Could you check a few things on this model? Use its own coordinates, in mm. A direction names the side the tool comes from. Coordinates: 2 decimals unless noted, no trailing zeros. Write each loop counter-clockwise with the first axis right and the second up, starting at its lowest first coordinate (ties: lowest second). Pieces come first, ordered by that corner, then holes. Notation, with made-up numbers: (36, -34) - (71, -34) arc R30 ccw to (71, 2) - close; hole circle Ø2 at (60.25, 39). An arc over 180 degrees is marked (long way). Answer as a JSON object with one key per item and string values. Group by question number.
1) On a 3-axis mill with a long thin cutter (end or side, diameter ignored), from which of +Z, -Z, +X, -X, +Y, -Y can I reach the whole of each face in a straight line? I mean faces 4 (the flat face through (0, -19, 12)), 5 (the flat face through (19, 0, 12)), 6 (the flat face through (-19, 0, 12)), 7 (the flat face through (0, 19, 12)), 8 (the cylindrical face through (-6, 0, 5)). Say none if no direction works.
2) Please list where these lines run through material, in increasing order: line 1 along Y through (x, z) = (0, 7.5); line 2 along X through (y, z) = (5.5, 4.75); line 3 along X through (y, z) = (4, 5.25).
3) If we section it at C-C (z = 5): Write out the boundary of the cut face in (x, y), plus the area to 3 significant figures.
4) Will these pins go through, and if not, where does the flat tip stop? pin 1 Ø1.2 at (x, z) = (-8, 11.5) entering from -Y; pin 2 Ø1.5 at (x, z) = (3.5, 11) entering from +Y; pin 3 Ø2 at (y, z) = (-0.5, 12) entering from +X.
5) If we section it at D-D (x = -7): Write out the boundary of the cut face in (y, z).
6) We'd pull the mould along Y, two halves only. Please class faces 1 (the flat face through (0, 0, 10)), 2 (the flat face through (0, 21, 5)), 3 (the flat face through (0, -21, 5)): released by +Y, released by -Y, zero draft, split by the parting line, or undercut.
7) If we section it at A-A (y = 0): Write out the boundary of the cut face in (x, z), plus the area to 3 significant figures.
```python
from build123d import *

# Parameters (mm, degrees)
SKETCH_W     = 42
SKETCH_H     = 42
SKETCH_R     = 6
PAD_DEPTH    = 10
SKETCH001_W  = 38
SKETCH001_H  = 38
PAD001_DEPTH = 4


with BuildPart() as part:
    # Sketch → Pad (new body)
    with BuildSketch(Plane.XY):
        Rectangle(SKETCH_W, SKETCH_H)
        Circle(SKETCH_R, mode=Mode.SUBTRACT)
    extrude(amount=PAD_DEPTH)

    # Sketch001 (on Face7 of Pad) → Pad001 (join)
    with BuildSketch(Plane.XY.offset(10)):
        Rectangle(SKETCH001_W, SKETCH001_H)
    extrude(amount=PAD001_DEPTH)


solid = part.part
```
Here are the results:
{
 "1": {"face 4": "+Z, +X, -X, -Y", "face 5": "+Z, +X, +Y, -Y", "face 6": "+Z, -X, +Y, -Y", "face 7": "+Z, +X, -X, +Y", "face 8": "-Z"},
 "2": {"line 1": "y = -21 to -6, 6 to 21", "line 2": "x = -21 to -2.4, 2.4 to 21", "line 3": "x = -21 to -4.47, 4.47 to 21"},
 "3": {"outline": "(-21, -21) - (21, -21) - (21, 21) - (-21, 21) - close; hole circle Ø12 at (0, 0)", "area": "1,650 mm²"},
 "4": {"pin 1": "stops at y = -19", "pin 2": "stops at y = 19", "pin 3": "stops at x = 19"},
 "5": {"outline": "(-21, 0) - (21, 0) - (21, 10) - (19, 10) - (19, 14) - (-19, 14) - (-19, 10) - (-21, 10) - close"},
 "6": {"face 1": "undercut", "face 2": "released by +Y", "face 3": "released by -Y"},
 "7": {"outline": "(-21, 0) - (-6, 0) - (-6, 10) - (6, 10) - (6, 0) - (21, 0) - (21, 10) - (19, 10) - (19, 14) - (-19, 14) - (-19, 10) - (-21, 10) - close", "area": "452 mm²"}
}
